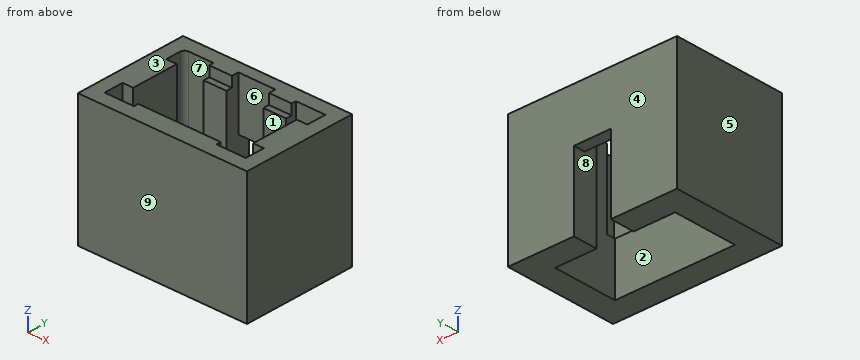
from build123d import *

# Parameters (mm, degrees)
SKETCH1_W               = 18.25
SKETCH1_H               = 12.3
SKETCH1_W_2             = 14.25
SKETCH1_H_2             = 8.3
BOSS_EXTRUDE1_DEPTH     = 14
SKETCH4_W               = 8.9
SKETCH4_H               = 0.65
BOSS_EXTRUDE2_DEPTH     = 12.9
SKETCH4_3_W             = 0.65
SKETCH4_3_H             = 5.1
BOSS_EXTRUDE3_DEPTH     = 14
SKETCH5_W               = 4
SKETCH5_H               = 2.65
CUT_EXTRUDE2_DEPTH      = 8.3
BOSS_EXTRUDE4_DEPTH     = 5.65
SKETCH7_W               = 4
SKETCH7_H               = 1.4
CUT_EXTRUDE3_DEPTH      = 6.7
SKETCH8_R               = 0.5
CUT_EXTRUDE4_DEPTH      = 8.35
MIRROR2_COPY_1_SKETCH_R = 0.5
MIRROR2_COPY_1_DEPTH    = 8.35
CUT_EXTRUDE5_DEPTH      = 8.35


with BuildPart() as part:
    # Sketch1 → Boss-Extrude1 (new body)
    with BuildSketch(Plane.XY):
        Rectangle(SKETCH1_W, SKETCH1_H)
        Rectangle(SKETCH1_W_2, SKETCH1_H_2, mode=Mode.SUBTRACT)
    extrude(amount=BOSS_EXTRUDE1_DEPTH)

    # Sketch4 → Boss-Extrude2 (add)
    with BuildSketch(Plane(origin=(0, 0, 0), x_dir=(-1, 0, 0), z_dir=(0, 0, -1))):
        with Locations((0, 3.825)):
            Rectangle(SKETCH4_W, SKETCH4_H)
        with Locations((0, -3.825)):
            Rectangle(SKETCH4_W, SKETCH4_H)
    extrude(amount=-BOSS_EXTRUDE2_DEPTH)

    # Sketch4<3> → Boss-Extrude3 (add)
    with BuildSketch(Plane(origin=(0, 0, 0), x_dir=(-1, 0, 0), z_dir=(0, 0, -1))):
        with Locations((-6.8, 0)):
            Rectangle(SKETCH4_3_W, SKETCH4_3_H)
        with Locations((6.8, 0)):
            Rectangle(SKETCH4_3_W, SKETCH4_3_H)
    extrude(amount=-BOSS_EXTRUDE3_DEPTH)

    # Sketch5 → Cut-Extrude2 (cut)
    with BuildSketch(Plane(origin=(0, 0, 0), x_dir=(-1, 0, 0), z_dir=(0, 0, -1))):
        with Locations((0, 4.825)):
            Rectangle(SKETCH5_W, SKETCH5_H)
    extrude(amount=-CUT_EXTRUDE2_DEPTH, mode=Mode.SUBTRACT)

    # Sketch6 → Boss-Extrude4 (add)
    with BuildSketch(Plane(origin=(0, 0, 0), x_dir=(-1, 0, 0), z_dir=(0, 0, -1))):
        Polygon((6.475, -3.5), (4.45, -3.5), (4.45, -4.15), (7.125, -4.15), (7.125, -2.55), (6.475, -2.55), align=None)
        Polygon((6.475, 3.5), (6.475, 2.55), (7.125, 2.55), (7.125, 4.15), (4.45, 4.15), (4.45, 3.5), align=None)
        Polygon((-7.125, 2.55), (-6.475, 2.55), (-6.475, 3.5), (-4.45, 3.5), (-4.45, 4.15), (-7.125, 4.15), align=None)
        Polygon((-4.45, -4.15), (-4.45, -3.5), (-6.475, -3.5), (-6.475, -2.55), (-7.125, -2.55), (-7.125, -4.15), align=None)
    extrude(amount=-BOSS_EXTRUDE4_DEPTH)

    # Sketch7 → Cut-Extrude3 (cut, through all)
    with BuildSketch(Plane(origin=(0, 0, 8.3), x_dir=(-1, 0, 0), z_dir=(0, 0, -1))):
        with Locations((0, 4.2)):
            Rectangle(SKETCH7_W, SKETCH7_H)
    extrude(amount=-CUT_EXTRUDE3_DEPTH, mode=Mode.SUBTRACT)

    # Sketch8 → Cut-Extrude4 (cut)
    with BuildSketch(Plane.XY.offset(14)):
        with Locations((-7.125, 4.15)):
            Circle(SKETCH8_R)
    cut_extrude4 = extrude(amount=-CUT_EXTRUDE4_DEPTH, mode=Mode.SUBTRACT)

    # Mirror1: Cut-Extrude4 across plane
    add(cut_extrude4.mirror(Plane.ZX), mode=Mode.SUBTRACT)

    # Mirror2: Cut-Extrude4 across plane
    add(cut_extrude4.mirror(Plane(origin=(0, 0, 0), x_dir=(0, 0, 1), z_dir=(1, 0, 0))), mode=Mode.SUBTRACT)

    # Mirror2 copy 1 sketch → Mirror2 copy 1 (cut)
    with BuildSketch(Plane(origin=(0, 0, 14), x_dir=(-1, 0, 0), z_dir=(0, 0, 1))):
        with Locations((-7.125, 4.15)):
            Circle(MIRROR2_COPY_1_SKETCH_R)
    extrude(amount=-MIRROR2_COPY_1_DEPTH, mode=Mode.SUBTRACT)

    # Sketch9 → Cut-Extrude5 (cut)
    with BuildSketch(Plane.XY.offset(14)):
        with BuildLine():
            ThreePointArc((-7.625, -4.15), (-7.478553391, -4.503553391), (-7.125, -4.65))
            ThreePointArc((-7.125, -4.65), (-6.771446609, -4.503553391), (-6.625, -4.15))
            Line((-6.625, -4.15), (-4.45, -4.15))
            Line((-4.45, -4.15), (-4.45, -2.55))
            Line((-4.45, -2.55), (-6.475, -2.55))
            Line((-6.475, -2.55), (-7.125, -2.55))
            Line((-7.125, -2.55), (-7.125, -3.65))
            ThreePointArc((-7.125, -3.65), (-7.478553391, -3.796446609), (-7.625, -4.15))
        make_face()
        with BuildLine():
            ThreePointArc((-6.625, -4.15), (-6.771446609, -4.503553391), (-7.125, -4.65))
            Line((-7.125, -4.65), (-4.45, -4.65))
            Line((-4.45, -4.65), (-4.45, -4.15))
            Line((-4.45, -4.15), (-6.625, -4.15))
        make_face()
        with BuildLine():
            Line((-7.625, -2.55), (-7.625, -4.15))
            ThreePointArc((-7.625, -4.15), (-7.478553391, -3.796446609), (-7.125, -3.65))
            Line((-7.125, -3.65), (-7.125, -2.55))
            Line((-7.125, -2.55), (-7.625, -2.55))
        make_face()
        with BuildLine():
            Line((-7.625, 4.15), (-7.625, 2.55))
            Line((-7.625, 2.55), (-7.125, 2.55))
            Line((-7.125, 2.55), (-7.125, 3.65))
            ThreePointArc((-7.125, 3.65), (-7.478553391, 3.796446609), (-7.625, 4.15))
        make_face()
        with BuildLine():
            Line((-4.45, 4.65), (-7.125, 4.65))
            ThreePointArc((-7.125, 4.65), (-6.771446609, 4.503553391), (-6.625, 4.15))
            Line((-6.625, 4.15), (-4.45, 4.15))
            Line((-4.45, 4.15), (-4.45, 4.65))
        make_face()
        with BuildLine():
            ThreePointArc((7.125, -3.65), (7.478553391, -3.796446609), (7.625, -4.15))
            Line((7.625, -4.15), (7.625, -2.55))
            Line((7.625, -2.55), (7.125, -2.55))
            Line((7.125, -2.55), (7.125, -3.65))
        make_face()
        with BuildLine():
            Line((6.625, -4.15), (4.45, -4.15))
            Line((4.45, -4.15), (4.45, -4.65))
            Line((4.45, -4.65), (7.125, -4.65))
            ThreePointArc((7.125, -4.65), (6.771446609, -4.503553391), (6.625, -4.15))
        make_face()
        with BuildLine():
            Line((4.45, -2.55), (4.45, -4.15))
            Line((4.45, -4.15), (6.625, -4.15))
            ThreePointArc((6.625, -4.15), (6.771446609, -4.503553391), (7.125, -4.65))
            ThreePointArc((7.125, -4.65), (7.478553391, -4.503553391), (7.625, -4.15))
            ThreePointArc((7.625, -4.15), (7.478553391, -3.796446609), (7.125, -3.65))
            Line((7.125, -3.65), (7.125, -2.55))
            Line((7.125, -2.55), (6.475, -2.55))
            Line((6.475, -2.55), (4.45, -2.55))
        make_face()
        with BuildLine():
            ThreePointArc((7.625, -4.15), (7.478553391, -4.503553391), (7.125, -4.65))
            Line((7.125, -4.65), (7.625, -4.65))
            Line((7.625, -4.65), (7.625, -4.15))
        make_face()
        with BuildLine():
            Line((7.625, 4.65), (7.125, 4.65))
            ThreePointArc((7.125, 4.65), (7.478553391, 4.503553391), (7.625, 4.15))
            Line((7.625, 4.15), (7.625, 4.65))
        make_face()
        with BuildLine():
            Line((7.625, 2.55), (7.625, 4.15))
            ThreePointArc((7.625, 4.15), (7.478553391, 3.796446609), (7.125, 3.65))
            Line((7.125, 3.65), (7.125, 2.55))
            Line((7.125, 2.55), (7.625, 2.55))
        make_face()
        with BuildLine():
            Line((7.125, 4.65), (4.45, 4.65))
            Line((4.45, 4.65), (4.45, 4.15))
            Line((4.45, 4.15), (6.625, 4.15))
            ThreePointArc((6.625, 4.15), (6.771446609, 4.503553391), (7.125, 4.65))
        make_face()
        with BuildLine():
            Line((6.625, 4.15), (4.45, 4.15))
            Line((4.45, 4.15), (4.45, 2.55))
            Line((4.45, 2.55), (6.475, 2.55))
            Line((6.475, 2.55), (7.125, 2.55))
            Line((7.125, 2.55), (7.125, 3.65))
            ThreePointArc((7.125, 3.65), (7.478553391, 3.796446609), (7.625, 4.15))
            ThreePointArc((7.625, 4.15), (7.478553391, 4.503553391), (7.125, 4.65))
            ThreePointArc((7.125, 4.65), (6.771446609, 4.503553391), (6.625, 4.15))
        make_face()
        with BuildLine():
            Line((-7.625, -4.15), (-7.625, -4.65))
            Line((-7.625, -4.65), (-7.125, -4.65))
            ThreePointArc((-7.125, -4.65), (-7.478553391, -4.503553391), (-7.625, -4.15))
        make_face()
    extrude(amount=-CUT_EXTRUDE5_DEPTH, mode=Mode.SUBTRACT)


solid = part.part
CAD build for the part. Positions are in the model's coordinates, mm. Face numbers are marked on the shaded views. A direction names the side the tool comes from. Give positions to 0.01 mm unless a question says otherwise; leave off trailing zeros. Loops run counter-clockwise (first coordinate to the right, second up) from the corner with the lowest first, then second, coordinate; pieces in that order, holes last. Notation, with made-up numbers: M 78,-3.5 L 130,-3.5 A29 cw 130,33.5 Z; hole C 57,24 d6. An arc over 180 degrees is marked long. Write each question's results on one line, items separated by ' | '.
Q1. Band-saw the part on A-A on y = 3.25. Write the cut outline in (x, z) (3 decimals), and give its area (3 significant figures).
Geometry check:
outline: M -9.125,0 L -6.475,0 L -6.475,5.65 L -7.625,5.65 L -7.625,14 L -9.125,14 Z; M 6.475,0 L 9.125,0 L 9.125,14 L 7.625,14 L 7.625,5.65 L 6.475,5.65 Z | area: 55.0 mm²
Q2. Which spindle directions (+Z, -Z, +X, -X, +Y, -Y) get a long thin tool onto all of the face, cutting with end or side? Do the marked faces 5, 6, 7, 8 and 9. Say none if no direction does.
Geometry check:
face 5: +Z, -Z, -X, +Y, -Y | face 6: +Z, -Z | face 7: +Z | face 8: -Z | face 9: +Z, -Z, +X, -X, -Y
Q3. Flat gauge pins, fed straight in: P1, Ø3, axis at x = -2.5, y = 1, coming from the -Z side; P2, Ø1.4, axis at x = 0.5, y = 5.5, coming from the -Z side; P3, Ø1.5, axis at x = -1.5, y = 3.5, coming from the +Z side. Where does each tip first touch, or does it go through?
Geometry check:
P1: passes through | P2: stops at z = 8.3 | P3: stops at z = 12.9
Q4. Band-saw the part on B-B on x = -3.75. Write the cut outline in (y, z), and give its area (3 significant figures).
Geometry check:
outline: M -6.15,0 L -3.5,0 L -3.5,12.9 L -4.15,12.9 L -4.15,14 L -6.15,14 Z; M 3.5,0 L 6.15,0 L 6.15,14 L 4.15,14 L 4.15,12.9 L 3.5,12.9 Z | area: 72.8 mm²
Q5. Mould opens along Y. For the marked faces 1, 2, 3 and 4 say: pulls with the +Y half, pulls with the -Y half, needs draft (parallel to the pull), parting line crosses it, or undercut.
Geometry check:
face 1: undercut | face 2: undercut | face 3: needs draft | face 4: pulls with the +Y half
Q6. Probe probe 1 along Y at (x, z) = (-7, 8.5); probe 2 along X at (y, z) = (-3, 6) (3 decimals); probe 3 along X at (y, z) = (3.75, 11.25) (3 decimals). List the from-to ranges inside material, lowest first.
Geometry check:
probe 1: y = -6.15 to -4.65, -2.55 to 2.55, 4.65 to 6.15 | probe 2: x = -9.125 to -7.625, 7.625 to 9.125 | probe 3: x = -9.125 to -7.625, -4.45 to -2, 2 to 4.45, 7.625 to 9.125
Q7. Band-saw the part on D-D on x = 7. Write the cut outline in (y, z), and give its area (3 significant figures).
Geometry check:
outline: M -6.15,0 L 6.15,0 L 6.15,14 L 4.65,14 L 4.65,5.65 L 2.55,5.65 L 2.55,14 L -2.55,14 L -2.55,5.65 L -4.65,5.65 L -4.65,14 L -6.15,14 Z | area: 137 mm²
